Here's the drawing with two shaded views (mm, measured from the low corner). I have some questions. Give positions to 0.01 mm unless a question says otherwise; leave off trailing zeros. Write each loop counter-clockwise with the first axis right and the second up, starting at its lowest first coordinate (ties: lowest second). Pieces come first, ordered by that corner, then holes. Notation, with made-up numbers: (56, 22.5) -> (103, 22.5) arc R17 cw to (103, 39.5) -> close; hole circle Ø6 at (82.25, 6). An arc over 180 degrees is marked (long way). One line per item, written item: value.
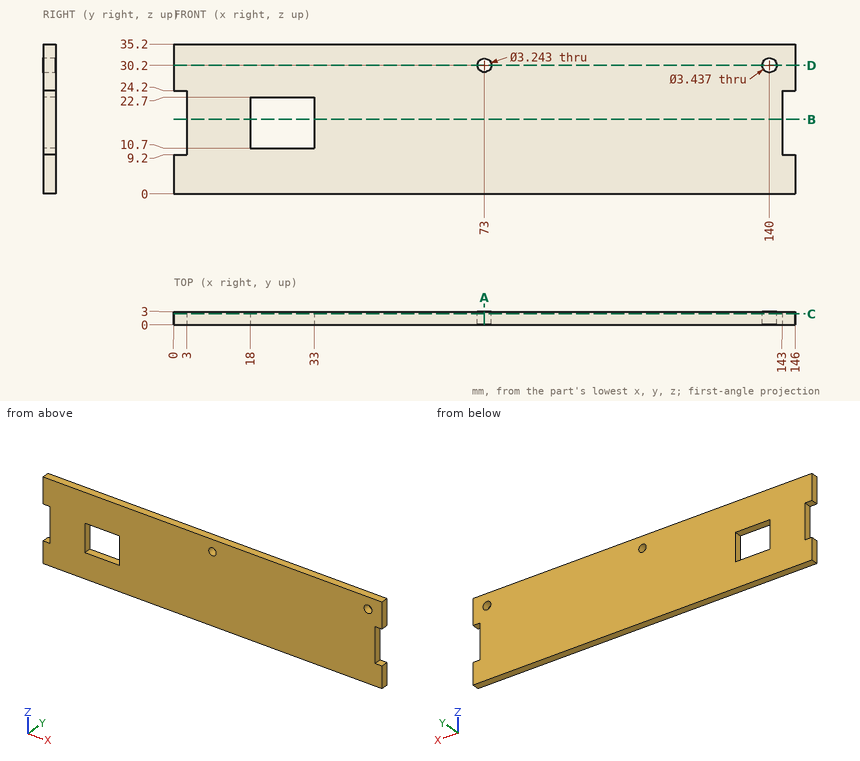
1) Will these pins go through, and if not, where does the flat tip stop? pin 1 (1.5 mm diameter, centred on y = 1, z = 17, fed in from -X); pin 2 (0.9 mm diameter, centred on y = 1.5, z = 17, fed in from +X).
Answer list:
pin 1: stops at x = 3
pin 2: stops at x = 143
2) I need wall thicknesses on L1, parallel to X at y = 1.9, z = 30.2; L2, parallel to Z at x = 73, y = 2.15; L3, parallel to Z at x = 140, y = 2.05. Which ranges of each line are inside material? Lowest first, please.
Answer list:
L1: x = 0 to 71.38, 74.62 to 138.28, 141.72 to 146
L2: z = 0 to 28.58, 31.82 to 35.2
L3: z = 0 to 28.48, 31.92 to 35.2
3) If we section it at A-A (x = 73): Write out the boundary of the cut face in (y, z).
Answer list:
outline: (0, 0) -> (3, 0) -> (3, 28.58) -> (0, 28.58) -> close; (0, 31.82) -> (3, 31.82) -> (3, 35.2) -> (0, 35.2) -> close
4) If we section it at C-C (y = 2.5): Write out the boundary of the cut face in (x, z).
Answer list:
outline: (0, 0) -> (146, 0) -> (146, 9.2) -> (143, 9.2) -> (143, 24.2) -> (146, 24.2) -> (146, 35.2) -> (0, 35.2) -> (0, 24.2) -> (3, 24.2) -> (3, 9.2) -> (0, 9.2) -> close; hole (18, 10.7) -> (33, 10.7) -> (33, 22.7) -> (18, 22.7) -> close; hole circle Ø3.24 at (73, 30.2); hole circle Ø3.44 at (140, 30.2)
5) If we section it at D-D (z = 30.2): Write out the boundary of the cut face in (x, y), and give its area (3 significant figures).
Answer list:
outline: (0, 0) -> (71.38, 0) -> (71.38, 3) -> (0, 3) -> close; (74.62, 0) -> (138.28, 0) -> (138.28, 3) -> (74.62, 3) -> close; (141.72, 0) -> (146, 0) -> (146, 3) -> (141.72, 3) -> close
area: 418 mm^2
6) If we section it at B-B (z = 17.5): Write out the boundary of the cut face in (x, y).
Answer list:
outline: (3, 0) -> (18, 0) -> (18, 3) -> (3, 3) -> close; (33, 0) -> (143, 0) -> (143, 3) -> (33, 3) -> close
